For this review, take the finished solid that the model builds, in its own axes (mm). A direction names the side the tool comes from. Coordinates: 2 decimals unless noted, no trailing zeros. Loops run counter-clockwise (first coordinate to the right, second up) from the corner with the lowest first, then second, coordinate; pieces in that order, holes last.
1. Machinability: for faces 1 (the face through (-0.33, -98.84, -7.493)), 2 (the face through (0, -7, 0)), which of the approach directions +Z, -Z, +X, -X, +Y, -Y give a long, thin tool a straight path to every point of the face, cutting with its end or side? Answer none if there is none.
2. Take a section at D-D, the plane y = -170. State the section outline as (x, z) points.
3. Take a section at C-C, the plane y = -124.5. State the section outline as (x, z) points.
4. Clearance check with flat-ended pins moving along their axes: P1, Ø5, axis at x = 11, y = -54, coming from the -Z side; P2, Ø1, axis at x = 0.5, z = 6, coming from the +Y side; P3, Ø12, axis at y = -94.5, z = -3, coming from the +X side; P4, Ø5, axis at x = -5, y = -105, coming from the +Z side. State where each tip first meets the part, or that it passes through.
5. To check wall thickness, follow probe 1 along Y at (x, z) = (-3, 0); probe 2 along Z at (x, y) = (6, -10); probe 3 along Y at (x, z) = (-4, -13). State the ranges of each line that lie inside material, in increasing order.
6. Mouldability with a two-part tool opening along Y and no side actions: class faces 3 (the face through (0, -180, 0)), 4 (the face through (0, 0, 0)), 5 (the face through (-10.4, -20, -6.3)) as pulls with the +Y half, pulls with the -Y half, needs draft (parallel to the pull), parting line crosses it, or undercut.
7. Take a section at A-A, the plane x = 0. Count the separate pieces of the cut face and the enclosed holes in it, then the cut area to 3 significant figures.
```python
from build123d import *

# Parameters (mm, degrees)
ESQUISSE2_R             = 3
ENL_V_MAT_EXTRU_1_DEPTH = 25


with BuildPart() as part:
    # Esquisse1 → Base-Révolution (revolve)
    with BuildSketch(Plane.XY, mode=Mode.PRIVATE) as base_r_volution_sk:
        with BuildLine():
            Line((0, 0), (-14, 0))
            Line((-14, 0), (-15, -1))
            Line((-15, -1), (-15, -19))
            Line((-15, -19), (-14, -20))
            Line((-14, -20), (-12, -20))
            ThreePointArc((-12, -20), (-10.585786438, -20.585786438), (-10, -22))
            Line((-10, -22), (-10, -36))
            Line((-10, -36), (-9.5, -36))
            ThreePointArc((-9.5, -36), (-8.085786438, -36.585786438), (-7.5, -38))
            Line((-7.5, -38), (-7.5, -158))
            ThreePointArc((-7.5, -158), (-8.085786438, -159.414213562), (-9.5, -160))
            Line((-9.5, -160), (-14, -160))
            Line((-14, -160), (-15, -161))
            Line((-15, -161), (-15, -179))
            Line((-15, -179), (-14, -180))
            Line((-14, -180), (0, -180))
            Line((0, -180), (0, 0))
        make_face()
    revolve(base_r_volution_sk.sketch.rotate(Axis((0, 0, 0), (0, -1, 0)), 270), axis=Axis((0, 0, 0), (0, -1, 0)))

    # Esquisse2 → Enlèv. mat.-Extru.1 (cut, symmetric)
    with BuildSketch(Plane(origin=(0, 0, 0), x_dir=(0, 0, -1), z_dir=(1, 0, 0))):
        with Locations((0, -10)):
            Circle(ESQUISSE2_R)
        with Locations((0, -170)):
            Circle(ESQUISSE2_R)
    extrude(amount=ENL_V_MAT_EXTRU_1_DEPTH, both=True, mode=Mode.SUBTRACT)


solid = part.part
```
Results list:
1. face 1: none
1. face 2: +X, -X
2. outline: (-14.7, -3) arc R15 ccw to (14.7, -3) - close; (-14.7, 3) - (14.7, 3) arc R15 ccw to start
3. outline: circle Ø15 at (0, 0)
4. P1: passes through
4. P2: stops at y = 0
4. P3: stops at x = 7.5
4. P4: stops at z = 7.07
5. probe 1: y = -180 to -173, -167 to -13, -7 to 0
5. probe 2: z = -13.75 to -3, 3 to 13.75
5. probe 3: y = -180 to -160, -20 to 0
6. face 3: pulls with the -Y half
6. face 4: pulls with the +Y half
6. face 5: undercut
7. separate pieces: 1
7. enclosed holes: 2
7. area: 3,320 mm2
